```python
from build123d import *

# Parameters (mm, degrees)
SKETCH_1_R          = 6
SKETCH_1_R_2        = 2.1
SKETCH_1_R_3        = 1.6
EXTRUDE_1_DEPTH     = 8
CUT_EXTRUDE_2_DEPTH = 71.670007783
FILLET_1_R          = 5


with BuildPart() as part:
    # 草图1 → 凸台-拉伸1 (new body)
    with BuildSketch(Plane(origin=(0, 0, 0), x_dir=(0, 0, -1), z_dir=(1, 0, 0))):
        with BuildLine():
            Line((-17.5, -47), (-17.5, -68))
            Line((-17.5, -68), (17.5, -68))
            Line((17.5, -68), (17.5, -47))
            Line((17.5, -47), (9.879034185, 1.550704218))
            ThreePointArc((9.879034185, 1.550704218), (6.75266911, 7.375734533), (0.675040765, 9.977189983))
            ThreePointArc((0.675040765, 9.977189983), (-1.314197069, 10.921876413), (-2.122447005, 12.970346978))
            Line((-2.122447005, 12.970346978), (-2.122447005, 37.772165508))
            Line((-2.122447005, 37.772165508), (-10.122447005, 37.772165508))
            Line((-10.122447005, 37.772165508), (-10.122447005, 0))
            Line((-10.122447005, 0), (-17.5, -47))
        make_face()
        Circle(SKETCH_1_R, mode=Mode.SUBTRACT)
        with Locations((-12.5, -50)):
            Circle(SKETCH_1_R_2, mode=Mode.SUBTRACT)
        with Locations((12.5, -50)):
            Circle(SKETCH_1_R_2, mode=Mode.SUBTRACT)
        with Locations((-12.5, -63)):
            Circle(SKETCH_1_R_2, mode=Mode.SUBTRACT)
        with Locations((12.5, -63)):
            Circle(SKETCH_1_R_2, mode=Mode.SUBTRACT)
        with Locations((-5.122447005, 34.772165508)):
            Circle(SKETCH_1_R_3, mode=Mode.SUBTRACT)
        with Locations((-5.122447005, 14.772165508)):
            Circle(SKETCH_1_R_3, mode=Mode.SUBTRACT)
    extrude(amount=EXTRUDE_1_DEPTH)

    # 草图3 → 切除-拉伸2 (cut, through all)
    with BuildSketch(Plane(origin=(8, 0, 0), x_dir=(0, 0, -1), z_dir=(1, 0, 0))):
        with BuildLine():
            Line((-6.920512772, -11.844929578), (-11.943527577, -43.844929578))
            ThreePointArc((-11.943527577, -43.844929578), (-11.715581533, -44.649972914), (-10.955624159, -45))
            Line((-10.955624159, -45), (10.955624159, -45))
            ThreePointArc((10.955624159, -45), (11.715581533, -44.649972914), (11.943527577, -43.844929578))
            Line((11.943527577, -43.844929578), (6.920512772, -11.844929578))
            ThreePointArc((6.920512772, -11.844929578), (6.582582268, -11.240042626), (5.932609354, -11))
            Line((5.932609354, -11), (-5.932609354, -11))
            ThreePointArc((-5.932609354, -11), (-6.582582268, -11.240042626), (-6.920512772, -11.844929578))
        make_face()
        with BuildLine():
            Line((-10.5, -55.196152423), (-10.5, -57.803847577))
            ThreePointArc((-10.5, -57.803847577), (-10.366025404, -58.303847577), (-10, -58.669872981))
            ThreePointArc((-10, -58.669872981), (-8.394106246, -60.146644697), (-7.569933514, -62.166666667))
            ThreePointArc((-7.569933514, -62.166666667), (-7.229417441, -62.763762616), (-6.583920217, -63))
            Line((-6.583920217, -63), (6.583920217, -63))
            ThreePointArc((6.583920217, -63), (7.229417441, -62.763762616), (7.569933514, -62.166666667))
            ThreePointArc((7.569933514, -62.166666667), (8.394106246, -60.146644697), (10, -58.669872981))
            ThreePointArc((10, -58.669872981), (10.366025404, -58.303847577), (10.5, -57.803847577))
            Line((10.5, -57.803847577), (10.5, -55.196152423))
            ThreePointArc((10.5, -55.196152423), (10.366025404, -54.696152423), (10, -54.330127019))
            ThreePointArc((10, -54.330127019), (8.394106246, -52.853355303), (7.569933514, -50.833333333))
            ThreePointArc((7.569933514, -50.833333333), (7.229417441, -50.236237384), (6.583920217, -50))
            Line((6.583920217, -50), (-6.583920217, -50))
            ThreePointArc((-6.583920217, -50), (-7.229417441, -50.236237384), (-7.569933514, -50.833333333))
            ThreePointArc((-7.569933514, -50.833333333), (-8.394106246, -52.853355303), (-10, -54.330127019))
            ThreePointArc((-10, -54.330127019), (-10.366025404, -54.696152423), (-10.5, -55.196152423))
        make_face()
    extrude(amount=-CUT_EXTRUDE_2_DEPTH, mode=Mode.SUBTRACT)

    # 圆角1
    fillet_1_edges = [part.edges().sort_by_distance(p)[0] for p in [
        (4, -47, -17.5),
        (4, -68, -17.5),
        (4, -68, 17.5),
        (4, -47, 17.5),
    ]]
    fillet(fillet_1_edges, radius=FILLET_1_R)


solid = part.part
```
Geometry: final body of the model. Coordinates: model frame, mm. A direction names the side the tool comes from. Coordinates: 2 decimals unless noted, no trailing zeros. Write each loop counter-clockwise with the first axis right and the second up, starting at its lowest first coordinate (ties: lowest second). Pieces come first, ordered by that corner, then holes. Notation, with made-up numbers: M 78,-22.5 L 109,-22.5 A21 cw 109,7.5 Z; hole C -16.5,-13 d7. An arc over 180 degrees is marked long. Answer as CSV lines item,"result". Start each with the question number.
Q1. Cut plane B-B on x = 1.25. Count the separate pieces of the cut face and the enclosed holes in it, then the cut area to 3 significant figures.
Q2. Cut plane C-C on y = -2. Return the cut outline in (x, z).
Q3. Pin query (flat end, axial travel): P1, Ø4, axis at x = 6, y = 6.5, coming from the +Z side; P2, Ø4, axis at x = 2.5, y = 26, coming from the -Z side; P3, Ø2, axis at x = 6, y = -15.5, coming from the -Z side. Return the tip coordinate at first contact, or that it passes through.
Q4. Reachability of faces 1 (the flat face through (4, -68, 0)), 2 (the flat face through (4.056, -28.069, -9.467)) from +Z, -Z, +X, -X, +Y, -Y: full face, straight path, thin tool, end or side. Return the list, or none.
Q5. Mould query, pull axis Z, two halves, no side actions, for faces 3 (the cylindrical face through (3.944, 7.312, -6.822)), 4 (the flat face through (4, 19, 10.122)), 5 (the flat face through (4.056, -27.621, 9.397)). Classes: released by +Z, released by -Z, zero draft, split by the parting line, or undercut.
Q6. Line query: line 1 (Y direction, x = 4.5, z = -5.5); line 2 (Y direction, x = 1, z = -1); line 3 (Y direction, x = 6, z = 5). Output: solid intervals per line, ascending. Write a range as from..to.
Q7. Cut plane A-A on y = -34.5. Return the cut outline in (x, z), then the cut area to 3 significant figures.
Findings below:
1,separate pieces,"1"
1,enclosed holes,"9"
1,area,"1,370 mm2"
2,outline,"M 0,-10.44 L 8,-10.44 L 8,-5.66 L 0,-5.66 Z; M 0,5.66 L 8,5.66 L 8,10.44 L 0,10.44 Z"
3,P1,"stops at z = 10.12"
3,P2,"stops at z = 2.12"
3,P3,"stops at z = -12.71"
4,face 1,"+Z, -Z, +X, -X, -Y"
4,face 2,"+X, -X"
5,face 3,"released by -Z"
5,face 4,"released by +Z"
5,face 5,"undercut"
6,line 1,"y = -68..-63, -50..-45, -11..-2.4, 2.4..8.35"
6,line 2,"y = -68..-63, -50..-45, -11..-5.92, 5.92..9.95"
6,line 3,"y = -68..-63, -50..-45, -11..-3.32, 3.32..13.18, 16.37..33.18, 36.37..37.77"
7,outline,"M 0,-15.54 L 8,-15.54 L 8,-10.48 L 0,-10.48 Z; M 0,10.48 L 8,10.48 L 8,15.54 L 0,15.54 Z"
7,area,"81.0 mm2"
